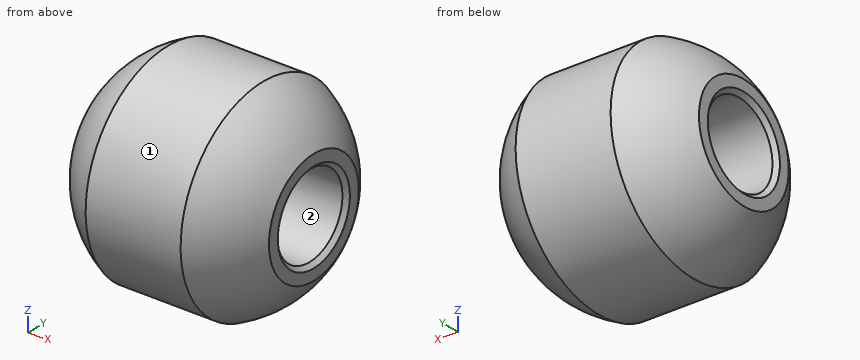
Autodesk Inventor part; units mm, degrees
ref_plane "YZ Plane" through (0, 0, 0) normal (1, 0, 0) x (0, 1, 0)
ref_plane "XZ Plane" through (0, 0, 0) normal (0, 1, 0) x (-1, 0, 0)
ref_plane "XY Plane" through (0, 0, 0) normal (0, 0, 1) x (1, 0, 0)
sketch "Sketch1" plane through (0, 0, 0) normal (0, 0, 1) x (1, 0, 0)
  line L0 (-4.7685, 2) -> (4.7685, 2)
  line L1 (4.7685, 2) -> (4.7685, 2.7408)
  line L2 (-4.7685, 2) -> (-4.7685, 2.7408)
  line L3 (0, 0) -> (2.529, 0)
  arc A0 (4.7685, 2.7408) -> (-4.7685, 2.7408) centre (0, 0) ccw
  dimension "d1" = 2
  dimension "d8" = 11
revolve "Revolution1" add sketch "Sketch1" angle 360 about axis through (0, 0, 0) along (1, 0, 0)
sketch "Sketch2" plane through (4.7685, 0, 0) normal (1, 0, 0) x (0, 0, -1)
  circle A0 centre (0, 0) radius 6
  circle A1 centre (0, 0) radius 2
  circle A2 centre (0, 0) radius 5
  dimension "d5" = 10
extrude "Extrusion1" cut sketch "Sketch2" against normal blind 10 contours A0
chamfer "Chamfer1" distance 0.2 angle 45 2 edges at (4.7685, -2, 0) (-4.7685, -2, 0)
equation "\"BendRadius\" = Thickness"
equation "\"BendReliefWidth\" = Thickness"
equation "\"BendReliefDepth\" = 0.5 * Thickness"
equation "\"CornerReliefSize\" = 4 * Thickness"
equation "\"MinimumRemnant\" = 2 * Thickness"
equation "\"TransitionRadius\" = BendRadius"
equation "\"JacobiRadiusSize\" = BendRadius"
equation "\"GapSize\" = Thickness"
properties part number "mắt trâu"
CAD build for the part. Positions are in the model's coordinates, mm. Face numbers are marked on the shaded views. Round coordinates to 2 decimals unless told otherwise and drop trailing zeros. Write each loop counter-clockwise with the first axis right and the second up, starting at its lowest first coordinate (ties: lowest second). Pieces come first, ordered by that corner, then holes. Notation, with made-up numbers: (-28.5, 73) -> (24.5, 73) arc R15 ccw to (24.5, 84) -> close; hole circle Ø5 at (-39, -24). An arc over 180 degrees is marked (long way). Answer as a JSON object with one key per item and string values.
(1) Band-saw the part on A-A, the plane y = 0. List the corners of the cut face in (x, z).
Reported:
{"outline": "(-4.77, -2.74) arc R5.5 ccw to (-2.29, -5) -> (2.29, -5) arc R5.5 ccw to (4.77, -2.74) -> (4.77, -2.2) -> (4.57, -2) -> (-4.57, -2) -> (-4.77, -2.2) -> close; (-4.77, 2.2) -> (-4.57, 2) -> (4.57, 2) -> (4.77, 2.2) -> (4.77, 2.74) arc R5.5 ccw to (2.29, 5) -> (-2.29, 5) arc R5.5 ccw to (-4.77, 2.74) -> close"}
(2) Pin check, flat tips, straight feed: P1, Ø3, axis at x = -0.5, y = 2, coming from the +Z side; P2, Ø1, axis at x = 3.5, z = -4, coming from the -Y side. Stop position of each tip, or through.
Reported:
{"P1": "stops at z = 4.97", "P2": "stops at y = -2.66"}
(3) Band-saw the part on D-D, the plane z = 4. List the corners of the cut face in (x, y) (3 decimals), then the cut area to 3 significant figures.
Reported:
{"outline": "(-2.291, -3) -> (2.291, -3) arc R3.775 ccw to (2.291, 3) -> (-2.291, 3) arc R3.775 ccw to start", "area": "39.9 mm^2"}
(4) Probe probe 1 along Z at (x, y) = (-0.5, 0); probe 2 along Z at (x, y) = (-4.5, 0); probe 3 along Y at (x, z) = (-3.75, -0.75). List the from-to ranges inside material, lowest first. Write a range as [from, to].
Reported:
{"probe 1": "z = [-5, -2], [2, 5]", "probe 2": "z = [-3.16, -2], [2, 3.16]", "probe 3": "y = [-3.95, -1.85], [1.85, 3.95]"}
(5) Band-saw the part on C-C, the plane x = 0.25. List the corners of the cut face in (y, z).
Reported:
{"outline": "circle Ø10 at (0, 0); hole circle Ø4 at (0, 0)"}
(6) Two-plate mould, pull along Z, no slides. Class the marked faces 1 and 2: +Z half, -Z half, draft (parallel to the pull), parting line (faces both ways), or undercut.
Reported:
{"face 1": "parting line", "face 2": "undercut"}
